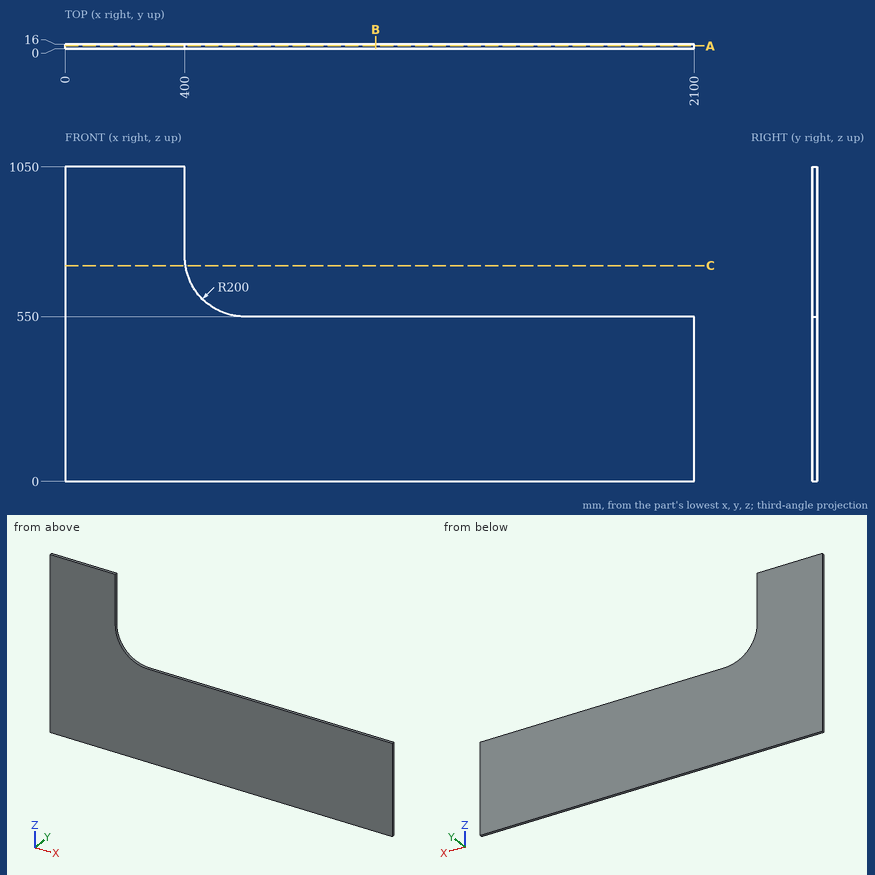
Source: three-view drawing plus pictorial views. Frame: mm from the lowest corner of the part. Coordinates: 2 decimals unless noted, no trailing zeros. Order: outer loops, then holes, each group sorted by start corner. A loop starts at its lowest first (then second) coordinate and runs counter-clockwise, first axis right, second up. Notation, with made-up numbers: (20.25, 88) -> (63.25, 88) arc R12 ccw to (63.25, 108) -> close; hole circle Ø7 at (1.5, -13). An arc over 180 degrees is marked (long way). Write item = value, one per line.
(1) Cut plane C-C on z = 720.5. Return loops of the section in (x, y), plus the area to 4 significant figures.
Solved:
outline = (0, 0) -> (402.19, 0) -> (402.19, 16) -> (0, 16) -> close
area = 6,435 mm²
(2) Cut plane A-A on y = 9.5. Return loops of the section in (x, z), plus the area to 3 significant figures.
Solved:
outline = (0, 0) -> (2100, 0) -> (2100, 550) -> (600, 550) arc R200 cw to (400, 750) -> (400, 1050) -> (0, 1050) -> close
area = 1,360,000 mm²
(3) Pin query (flat end, axial travel): pin 1 Ø4 at (x, y) = (1268.5, 7) entering from +Z; pin 2 Ø2 at (x, y) = (726, 6) entering from -Z; pin 3 Ø8 at (y, z) = (8, 953.5) entering from +X. Return the tip coordinate at first contact, or that it passes through.
Solved:
pin_1 = 550
pin_2 = 0
pin_3 = 400
(4) Cut plane B-B on x = 1037. Return loops of the section in (y, z).
Solved:
outline = (0, 0) -> (16, 0) -> (16, 550) -> (0, 550) -> close
(5) Line query: line 1 (Z direction, x = 1968.5, y = 3.75); line 2 (X direction, y = 9.5, z = 741); line 3 (X direction, y = 9.5, z = 704). Output: solid intervals per line, ascending.
Solved:
line_1 = 0 to 550
line_2 = 0 to 400.2
line_3 = 0 to 405.36
